```python
from build123d import *

# Parameters (mm, degrees)
SKETCH4_W          = 0.681153679
SKETCH4_H          = 0.530582866
CUT_EXTRUDE1_DEPTH = 0.3


with BuildPart() as part:
    # Sketch2 → Revolve2 (revolve)
    with BuildSketch(Plane.XY):
        with BuildLine():
            Line((-46, -4.2), (-46, -6.7))
            Line((-46, -6.7), (-46, -8.2))
            Line((-46, -8.2), (-54, -8.2))
            Line((-54, -8.2), (-54, -4.2))
            Line((-54, -4.2), (-53.041381265, -4.2))
            ThreePointArc((-53.041381265, -4.2), (-50, -6.7), (-46.958618735, -4.2))
            Line((-46.958618735, -4.2), (-46, -4.2))
        make_face()
    revolve(axis=Axis((0, 30.712444699, 0), (0, -1, 0)))

    # Sketch4 → Cut-Extrude1 (cut)
    with BuildSketch(Plane.XZ.offset(8.2)):
        Polygon((-49.606287717, 0), (-51.284076779, 0), (-51.284076779, -1.569276179), (-50.086680312, -1.569276179), (-50.086680312, -3.017624002), (-49.606287717, -3.017624002), (-49.606287717, -1.569276179), align=None)
        with Locations((-50.427257152, -0.658681261)):
            Rectangle(SKETCH4_W, SKETCH4_H, mode=Mode.SUBTRACT)
        Polygon((-47.068094007, 0), (-48.889283844, 0), (-48.889283844, -0.708871532), (-48.129259739, -0.708871532), (-48.889283844, -3.017624002), (-47.828118112, -3.017624002), (-47.068094007, -0.708871532), align=None)
    extrude(amount=-CUT_EXTRUDE1_DEPTH, mode=Mode.SUBTRACT)


solid = part.part
```
Here's how the part is built. I have some questions about the finished solid (model axes, mm). Give positions to 0.01 mm unless a question says otherwise; leave off trailing zeros. Loops run counter-clockwise (first coordinate to the right, second up) from the corner with the lowest first, then second, coordinate; pieces in that order, holes last. Notation, with made-up numbers: M -9.5,-7.5 L 29.5,-7.5 A23 ccw 29.5,1.5 Z; hole C 24.25,2.25 d3. An arc over 180 degrees is marked long. Return JSON: item names as keys, results as strings.
Item 1: Thinking about a two-plate mould opening in Z: for faces 1 (the flat face through (-36, -4.2, 40)), 2 (the cylindrical face through (5.99, -6.23, -45.61)), 3 (the cylindrical face through (11.706, -6.172, 52.716)), which applies, released by +Z, released by -Z, zero draft, split by the parting line, or undercut?
A:
{"face 1": "zero draft", "face 2": "undercut", "face 3": "split by the parting line"}
Item 2: Please list where these lines run through material, in increasing order: line 1 (X direction, y = -6, z = 0); line 2 (X direction, y = -6.35, z = 0); line 3 (Z direction, x = -15.5, y = -5.6).
A:
{"line 1": "x = -54 to -51.96, -48.04 to -46, 46 to 48.04, 51.96 to 54", "line 2": "x = -54 to -51.43, -48.57 to -46, 46 to 48.57, 51.43 to 54", "line 3": "z = -51.73 to -50.02, -45.04 to -43.31, 43.31 to 45.04, 50.02 to 51.73"}
Item 3: Imagine slicing it at B-B on y = -5.45. List the corners of the cut face in (x, z) for me, then the cut area to 3 significant figures.
A:
{"outline": "C 0,0 d108; C 0,0 d95.03; hole C 0,0 d104.97; hole C 0,0 d92", "area": "950 mm^2"}
Item 4: Imagine slicing it at A-A on x = 0. List the corners of the cut face in (y, z) for me.
A:
{"outline": "M -8.2,-54 L -4.2,-54 L -4.2,-53.04 A3.1 cw -4.2,-46.96 L -4.2,-46 L -8.2,-46 Z; M -8.2,46 L -4.2,46 L -4.2,46.96 A3.1 cw -4.2,53.04 L -4.2,54 L -8.2,54 Z"}
Item 5: I'm going to push flat-ended pins straight in: pin 1 Ø2 at (x, y) = (14, -7) entering from +Z; pin 2 Ø1 at (y, z) = (-6.5, 23) entering from -X; pin 3 Ø2 at (x, y) = (-41, -5.5) entering from +Z. Where does each tip first touch, or does it pass through?
A:
{"pin 1": "stops at z = 52.41", "pin 2": "stops at x = -49.09", "pin 3": "stops at z = 36.28"}
